For this review, take the finished solid that the model builds, in its own axes (mm). A direction names the side the tool comes from. Give positions to 0.01 mm unless a question says otherwise; leave off trailing zeros. Loops run counter-clockwise (first coordinate to the right, second up) from the corner with the lowest first, then second, coordinate; pieces in that order, holes last. Notation, with made-up numbers: (62.5, 17) -> (84.5, 17) arc R17 ccw to (84.5, 28) -> close; hole circle Ø1 at (-27, 20). An arc over 180 degrees is marked (long way). One line per question, with ' | ' between items. Start each with the question number.
(1) Consider section C-C (y = -6). Write out the cut boundary in (x, z).
(2) Draft analysis for pull direction Z (two halves, no side actions). For faces 1 (the cylindrical face through (-3.604, -4.93, 11.446)), 2 (the cylindrical face through (34.647, 9.86, -18.456)), 3 (the flat face through (-6, -10, 2)), state which applies: +Z half, -Z half, draft (parallel to the pull), parting line (faces both ways), or undercut.
(3) Consider section D-D (z = -16.5). Give the number of separate pieces and of enclosed holes in the cut face, and give its area (3 significant figures).
(4) Tool access review of faces 4 (the cylindrical face through (-16.69, 13.1, 28.47)), 5 (the cylindrical face through (-4.88, -4.56, 1.08)), 6 (the cylindrical face through (-34.594, 9.86, -18.759)), 7 (the cylindrical face through (-39.289, 15.966, 0.521)): name each direction out of +Z, -Z, +X, -X, +Y, -Y from which nothing blocks a thin tool from reaching the whole face with its end or side.
(5) Consider section B-B (y = 2.5). Write out the cut boundary in (x, z), and give its area (3 significant figures).
(6) Wall thickness on probe 1 along X at (y, z) = (2.45, 0); probe 2 along X at (y, z) = (17.5, -19.5); probe 3 along Y at (x, z) = (13.5, -1.5): over which ranges is each line inside the solid? List them lowest first.
(7) Consider section A-A (z = 0). Write out the cut boundary in (x, y).
(8) Insertion check: P1, Ø2, axis at x = 9, y = 0, coming from the +Z side; P2, Ø2, axis at x = -20.5, y = 3, coming from the -Z side; P3, Ø1, axis at x = -27, z = 15, coming from the -Y side. Each pin has a flat end and moves straight along its axis. Give the tip position at first contact, or say it passes through.
from build123d import *

# Parameters (mm, degrees)
SKETCH1_R           = 46
SKETCH1_R_2         = 3.5
BOSS_EXTRUDE1_DEPTH = 20
SKETCH2_R           = 33
CUT_EXTRUDE1_DEPTH  = 14
FILLET2_R           = 1
SKETCH3_R           = 12
BOSS_EXTRUDE2_DEPTH = 10
SKETCH4_R           = 2.5
CUT_EXTRUDE2_DEPTH  = 6
SKETCH5_R           = 5
CUT_EXTRUDE3_DEPTH  = 10
CHAMFER1_SIZE       = 1
SKETCH6_R           = 4
CUT_EXTRUDE4_DEPTH  = 69.058798176


with BuildPart() as part:
    # Sketch1 → Boss-Extrude1 (new body)
    with BuildSketch(Plane(origin=(0, 0, 0), x_dir=(1, 0, 0), z_dir=(0, 1, 0))):
        with Locations(Location((0, 0, 0), (0, 0, 270))):
            Circle(SKETCH1_R)
        with Locations(Location((0, 36, 0), (0, 0, 270))):
            Circle(SKETCH1_R_2, mode=Mode.SUBTRACT)
        with Locations(Location((-31.176914536, 18, 0), (0, 0, 270))):
            Circle(SKETCH1_R_2, mode=Mode.SUBTRACT)
        with Locations(Location((-31.176914536, -18, 0), (0, 0, 270))):
            Circle(SKETCH1_R_2, mode=Mode.SUBTRACT)
        with Locations(Location((0, -36, 0), (0, 0, 270))):
            Circle(SKETCH1_R_2, mode=Mode.SUBTRACT)
        with Locations(Location((31.176914536, -18, 0), (0, 0, 270))):
            Circle(SKETCH1_R_2, mode=Mode.SUBTRACT)
        with Locations(Location((31.176914536, 18, 0), (0, 0, 270))):
            Circle(SKETCH1_R_2, mode=Mode.SUBTRACT)
    extrude(amount=BOSS_EXTRUDE1_DEPTH)

    # Sketch2 → Cut-Extrude1 (cut)
    with BuildSketch(Plane(origin=(0, 20, 0), x_dir=(1, 0, 0), z_dir=(0, 1, 0))):
        Circle(SKETCH2_R)
    extrude(amount=-CUT_EXTRUDE1_DEPTH, mode=Mode.SUBTRACT)

    # Fillet2
    fillet2_edges = [part.edges().sort_by_distance(p)[0] for p in [
        (0, 0, -46),
    ]]
    fillet(fillet2_edges, radius=FILLET2_R)

    # Sketch3 → Boss-Extrude2 (add)
    with BuildSketch(Plane(origin=(0, 0, 0), x_dir=(-1, 0, 0), z_dir=(0, -1, 0))):
        with Locations(Location((0, 0, 0), (0, 0, 270))):
            Circle(SKETCH3_R)
    extrude(amount=BOSS_EXTRUDE2_DEPTH)

    # Sketch4 → Cut-Extrude2 (cut)
    with BuildSketch(Plane(origin=(0, 6, 0), x_dir=(1, 0, 0), z_dir=(0, 1, 0))):
        with Locations(Location((0, 0, 0), (0, 0, 270))):
            Circle(SKETCH4_R)
    extrude(amount=-CUT_EXTRUDE2_DEPTH, mode=Mode.SUBTRACT)

    # Sketch5 → Cut-Extrude3 (cut)
    with BuildSketch(Plane(origin=(0, -10, 0), x_dir=(-1, 0, 0), z_dir=(0, -1, 0))):
        with Locations(Location((0, 0, 0), (0, 0, 90))):
            Circle(SKETCH5_R)
    extrude(amount=-CUT_EXTRUDE3_DEPTH, mode=Mode.SUBTRACT)

    # Chamfer1
    chamfer1_edges = [part.edges().sort_by_distance(p)[0] for p in [
        (0, -10, 5),
    ]]
    chamfer(chamfer1_edges, length=CHAMFER1_SIZE)

    # Sketch6 → Cut-Extrude4 (cut, through all)
    with BuildSketch(Plane(origin=(0, 0, 0), x_dir=(0, 0, -1), z_dir=(1, 0, 0))):
        with Locations((0, 12)):
            Circle(SKETCH6_R)
    extrude(amount=-CUT_EXTRUDE4_DEPTH, mode=Mode.SUBTRACT)


solid = part.part
A:
1) outline: circle Ø24 at (0, 0); hole circle Ø10 at (0, 0)
2) face 1: parting line | face 2: undercut | face 3: draft
3) separate pieces: 3 | enclosed holes: 0 | area: 680 mm^2
4) face 4: +Y | face 5: -Y | face 6: +Y, -Y | face 7: -X
5) outline: circle Ø92 at (0, 0); hole circle Ø7 at (-31.18, -18); hole circle Ø7 at (-31.18, 18); hole circle Ø7 at (0, -36); hole circle Ø7 at (0, 36); hole circle Ø5 at (0, 0); hole circle Ø7 at (31.18, -18); hole circle Ø7 at (31.18, 18) | area: 6,400 mm^2
6) probe 1: x = -46 to -2.5, 2.5 to 46 | probe 2: x = -41.66 to -34.34, -28.01 to -26.62, 26.62 to 28.01, 34.34 to 41.66 | probe 3: y = 0 to 6
7) outline: (-46, 1) arc R1 ccw to (-45, 0) -> (-12, 0) -> (-12, -10) -> (-6, -10) -> (-5, -9) -> (-5, 0) -> (-2.5, 0) -> (-2.5, 6) -> (-33, 6) -> (-33, 8) -> (-46, 8) -> close; (-46, 16) -> (-33, 16) -> (-33, 20) -> (-46, 20) -> close; (2.5, 0) -> (5, 0) -> (5, -9) -> (6, -10) -> (12, -10) -> (12, 0) -> (45, 0) arc R1 ccw to (46, 1) -> (46, 20) -> (33, 20) -> (33, 6) -> (2.5, 6) -> close
8) P1: stops at z = 45.21 | P2: stops at z = -41.66 | P3: stops at y = 0
